from build123d import *

# Parameters (mm, degrees)
EXTRUDE_1_DEPTH      = 1.5
EXTRUDE_1_DEPTH_BACK = 1.5
SKETCH_1_W           = 116
SKETCH_1_H           = 15
SKETCH_1_R           = 1.75


with BuildPart() as part:
    # Sketch 1 → Extrude 1 (new, two sides: drawn at the far end of the back side and taken through both)
    with BuildSketch(Plane(origin=(0, 0, 0), x_dir=(1, 0, 0), z_dir=(0, 1, 0)).offset(-EXTRUDE_1_DEPTH_BACK)):
        Rectangle(SKETCH_1_W, SKETCH_1_H)
        with Locations(Location((53, 0, 0), (0, 0, 270))):
            Circle(SKETCH_1_R, mode=Mode.SUBTRACT)
        with Locations(Location((-53, 0, 0), (0, 0, 270))):
            Circle(SKETCH_1_R, mode=Mode.SUBTRACT)
        with Locations(Location((0, 0, 0), (0, 0, 270))):
            Circle(SKETCH_1_R, mode=Mode.SUBTRACT)
    extrude(amount=EXTRUDE_1_DEPTH + EXTRUDE_1_DEPTH_BACK)

    # Sketch 2 → Hole Wizard M3.51 (revolve, cut)
    with BuildSketch(Plane(origin=(0, 1.5, 0), x_dir=(0, 0, 1), z_dir=(1, 0, 0))):
        Polygon((0, 0), (0, 3), (1.95, 3), (1.95, 2.15), (4.1, 0), align=None)
    revolve(axis=Axis((0, 7.85, 0), (0, -1, 0)), mode=Mode.SUBTRACT)


solid = part.part
Work out the finished part from the listing and answer in its coordinate system (mm). Round coordinates to 2 decimals unless told otherwise and drop trailing zeros. Loops run counter-clockwise (first coordinate to the right, second up) from the corner with the lowest first, then second, coordinate; pieces in that order, holes last. Notation, with made-up numbers: (22.25, 0) - (34.25, 0) arc R17 cw to (34.25, 25) - close; hole circle Ø3 at (16, 6). An arc over 180 degrees is marked (long way). Use one line per item in the form item = value. Start each with the question number.
(1) Find section C-C on x = 0. Determine the outline of the cut face in (y, z).
(2) Find section A-A on x = -53. Determine the outline of the cut face in (y, z), and give its area (3 significant figures).
(3) Consider line 1 (X direction, y = -1.25, z = 0); line 2 (X direction, y = -0.15, z = 0); line 3 (X direction, y = 0.2, z = 2). Determine where each line is inside the solid, lowest interval first.
(4) Determine the mould class of faces 1 (the face through (-54.71, -0.02, -0.38)), 2 (the face through (-1, 1.5, -5)), 3 (the face through (58, 0, 0)) for opening direction X: +X half, -X half, draft (parallel to the pull), parting line (faces both ways), or undercut.
(5) Find section B-B on y = 0.45. Determine the outline of the cut face in (x, z).
Answer list:
q1.outline = (-1.5, -7.5) - (1.5, -7.5) - (1.5, -4.1) - (-0.65, -1.95) - (-1.5, -1.95) - close; (-1.5, 1.95) - (-0.65, 1.95) - (1.5, 4.1) - (1.5, 7.5) - (-1.5, 7.5) - close
q2.outline = (-1.5, -7.5) - (1.5, -7.5) - (1.5, -1.75) - (-1.5, -1.75) - close; (-1.5, 1.75) - (1.5, 1.75) - (1.5, 7.5) - (-1.5, 7.5) - close
q2.area = 34.5 mm^2
q3.line_1 = -58 to -54.75, -51.25 to -1.95, 1.95 to 51.25, 54.75 to 58
q3.line_2 = -58 to -54.75, -51.25 to -2.45, 2.45 to 51.25, 54.75 to 58
q3.line_3 = -58 to -1.96, 1.96 to 58
q4.face_1 = undercut
q4.face_2 = draft
q4.face_3 = +X half
q5.outline = (-58, -7.5) - (58, -7.5) - (58, 7.5) - (-58, 7.5) - close; hole circle Ø3.5 at (-53, 0); hole circle Ø6.1 at (0, 0); hole circle Ø3.5 at (53, 0)
